```python
from build123d import *

# Parameters (mm, degrees)
F0_R     = 40.1427902356
F1_DEPTH = 144.426420331
F1_TAPER = -3
F2_T     = -2.54
F3_R     = 0.254


with BuildPart() as f1:
    # F0 (on Top) → F1 (new body)
    with BuildSketch(Plane.XY):
        Circle(F0_R)
    extrude(amount=F1_DEPTH, taper=F1_TAPER)

    # F2
    f2_openings = [f1.faces().sort_by_distance(p)[0] for p in [
        (0, 0, 144.42642),
    ]]
    offset(amount=F2_T, openings=f2_openings, kind=Kind.INTERSECTION)

    # F3
    f3_edges = [f1.edges().sort_by_distance(p)[0] for p in [
        (-47.711858, 0, 144.42642),
        (-45.168372, 0, 144.42642),
    ]]
    fillet(f3_edges, radius=F3_R)


solid = f1.part
```
The model under review builds one solid part; all positions refer to its coordinate system, in mm. A direction names the side the tool comes from. Give positions to 0.01 mm unless a question says otherwise; leave off trailing zeros. Write each loop counter-clockwise with the first axis right and the second up, starting at its lowest first coordinate (ties: lowest second). Pieces come first, ordered by that corner, then holes. Notation, with made-up numbers: M 19.5,-28 L 37.5,-28 A17 cw 37.5,2 Z; hole C 63.5,24 d7. An arc over 180 degrees is marked long. Write each question's results on one line, items separated by ' | '. Start each with the question number.
1. We need section A-A (x = 0). Write out the cut boundary in (y, z).
2. We need section C-C (z = 83). Write out the cut boundary in (x, y), and give its area (3 significant figures).
3. For probe 1 along Z at (x, y) = (0, -26); probe 2 along Y at (x, z) = (-39, 120); probe 3 along X at (y, z) = (-27, 129), list the stretches that pass through material, from the lowest coordinate up. Write a range as [from, to].
4. For faces 4 (the flat face through (3.3, -45.5, 144.426)), 5 (the flat face through (-1, 1, 2.54)), list the 3-axis set-ups (+Z, -Z, +X, -X, +Y, -Y) from which the entire face can be reached by the end or side of a thin tool; tool diameter is ignored.
5. Insertion check: pin 1 Ø8 at (y, z) = (-34, 15) entering from +X; pin 2 Ø1.5 at (x, y) = (28.5, -9) entering from +Z; pin 3 Ø1 at (y, z) = (-31.5, 113.5) entering from +X. Each pin has a flat end and moves straight along its axis. Give the tip position at first contact, or say it passes through.
6. We need section B-B (z = 60). Write out the cut boundary in (x, y), and give its area (3 significant figures).
7. Mouldability with a two-part tool opening along X and no side actions: class faces 1 (the conical face through (-9.53, -42.93, 73.09)), 2 (the conical face through (-5.402, 41.143, 74.354)), 3 (the flat face through (-1, 1, 0)) as released by +X, released by -X, zero draft, split by the parting line, or undercut.
Results found:
1) outline: M -47.7,144.16 L -40.14,0 L 40.14,0 L 47.7,144.16 A0.25 ccw 47.44,144.43 L 45.41,144.43 A0.25 ccw 45.16,144.19 L 37.73,2.54 L -37.73,2.54 L -45.16,144.19 A0.25 ccw -45.41,144.43 L -47.44,144.43 A0.25 ccw Z
2) outline: C 0,0 d88.99; hole C 0,0 d83.9 | area: 691 mm^2
3) probe 1: z = [0, 2.54] | probe 2: y = [-25.2, -20.13], [20.13, 25.2] | probe 3: x = [-38.35, -35.2], [35.2, 38.35]
4) face 4: +Z, +X, -X, +Y, -Y | face 5: +Z
5) pin 1: stops at x = 27.85 | pin 2: stops at z = 2.54 | pin 3: stops at x = 34.11
6) outline: C 0,0 d86.57; hole C 0,0 d81.49 | area: 671 mm^2
7) face 1: split by the parting line | face 2: undercut | face 3: zero draft
